```python
from build123d import *

# Parameters (mm, degrees)
F0_R     = 1.5875
F1_DEPTH = 3.048


# Not quite as in the source:
# - a feature names something its author has since deleted; it is built from what else it names


with BuildPart() as f1:
    # F0 (on Front) → F1 (new body)
    with BuildSketch(Plane.XZ):
        with BuildLine():
            Line((-35.5894761368, 60.4198244451), (-34.9866182967, 55.8428987828))
            ThreePointArc((-34.9866182967, 55.8428987828), (-34.9404170511, 56.3828619929), (-34.925, 56.9245788358))
            ThreePointArc((-34.925, 56.9245788358), (-35.092593447, 58.7035019936), (-35.5894761368, 60.4198244451))
        make_face()
        with BuildLine():
            Line((-60.2004882138, 4.1402033601), (-60.2004882138, 8.1089543114))
            ThreePointArc((-60.2004882138, 8.1089543114), (-60.325, 6.1245788358), (-60.2004882138, 4.1402033601))
        make_face()
        with BuildLine():
            ThreePointArc((-34.9866182967, 55.8428987828), (-38.1087610636, 49.8172365933), (-44.45, 47.3995788358))
            Line((-44.45, 47.3995788358), (-44.45, 21.9995788358))
            ThreePointArc((-44.45, 21.9995788358), (-33.9832619763, 18.0603662058), (-28.7109436839, 8.1976758617))
            Line((-28.7109436839, 8.1976758617), (-34.9866182967, 55.8428987828))
        make_face()
        with BuildLine():
            ThreePointArc((-44.45, -9.7504211642), (-54.950325336, -5.7816713228), (-60.2004882138, 4.1402033601))
            Line((-60.2004882138, 4.1402033601), (-54.5067664898, -58.2925744899))
            ThreePointArc((-54.5067664898, -58.2925744899), (-51.9079352447, -50.5666823428), (-44.45, -47.276920164))
            Line((-44.45, -47.276920164), (-44.45, -9.7504211642))
        make_face()
        with BuildLine():
            ThreePointArc((-34.3514989997, -57.3754211642), (-37.3092814629, -50.2347026271), (-44.45, -47.276920164))
            Line((-44.45, -47.276920164), (-44.45, -54.2004211642))
            ThreePointArc((-44.45, -54.2004211642), (-42.2049359697, -55.130357134), (-41.275, -57.3754211642))
            Line((-41.275, -57.3754211642), (-34.3514989997, -57.3754211642))
        make_face()
        with BuildLine():
            Line((-44.45, 21.9995788358), (-44.45, 47.3995788358))
            ThreePointArc((-44.45, 47.3995788358), (-51.5919689055, 50.6223645302), (-53.9009645367, 58.1098612184))
            Line((-53.9009645367, 58.1098612184), (-60.2004882138, 8.1089543114))
            ThreePointArc((-60.2004882138, 8.1089543114), (-54.950325336, 18.0308289943), (-44.45, 21.9995788358))
        make_face()
        with Locations((-48.8420496888, 42.732682374)):
            Circle(F0_R, mode=Mode.SUBTRACT)
        with BuildLine():
            ThreePointArc((-28.7109436839, 8.1976758617), (-33.9832619763, 18.0603662058), (-44.45, 21.9995788358))
            Line((-44.45, 21.9995788358), (-44.45, 9.1638046543))
            ThreePointArc((-44.45, 9.1638046543), (-42.3009428141, 8.2736360216), (-41.4107741814, 6.1245788358))
            ThreePointArc((-41.4107741814, 6.1245788358), (-42.3009428141, 3.9755216499), (-44.45, 3.0853530172))
            Line((-44.45, 3.0853530172), (-44.45, -9.7504211642))
            ThreePointArc((-44.45, -9.7504211642), (-34.1131196636, -5.9238455389), (-28.7595280627, 3.7111341226))
            ThreePointArc((-28.7595280627, 3.7111341226), (-28.6211992399, 4.91433444), (-28.575, 6.1245788358))
            ThreePointArc((-28.575, 6.1245788358), (-28.6090223784, 7.1633535905), (-28.7109436839, 8.1976758617))
        make_face()
        with BuildLine():
            ThreePointArc((-53.9009645367, 58.1098612184), (-51.5919689055, 50.6223645302), (-44.45, 47.3995788358))
            ThreePointArc((-44.45, 47.3995788358), (-38.1087610636, 49.8172365933), (-34.9866182967, 55.8428987828))
            Line((-34.9866182967, 55.8428987828), (-35.5894761368, 60.4198244451))
            ThreePointArc((-35.5894761368, 60.4198244451), (-45.6421147488, 66.37468399), (-53.9009645367, 58.1098612184))
        make_face()
        with BuildLine():
            ThreePointArc((-41.275, 56.9245788358), (-42.2049359697, 54.6795148055), (-44.45, 53.7495788358))
            ThreePointArc((-44.45, 53.7495788358), (-46.6950640303, 59.169642866), (-41.275, 56.9245788358))
        make_face(mode=Mode.SUBTRACT)
        with BuildLine():
            Line((-44.45, 9.1638046543), (-44.45, 21.9995788358))
            ThreePointArc((-44.45, 21.9995788358), (-54.950325336, 18.0308289943), (-60.2004882138, 8.1089543114))
            Line((-60.2004882138, 8.1089543114), (-60.2004882138, 4.1402033601))
            ThreePointArc((-60.2004882138, 4.1402033601), (-54.950325336, -5.7816713228), (-44.45, -9.7504211642))
            Line((-44.45, -9.7504211642), (-44.45, 3.0853530172))
            ThreePointArc((-44.45, 3.0853530172), (-47.4892258186, 6.1245788358), (-44.45, 9.1638046543))
        make_face()
        with BuildLine():
            Line((-7.9375, -57.3754211642), (-34.3514989997, -57.3754211642))
            ThreePointArc((-34.3514989997, -57.3754211642), (-36.803283354, -63.9714386739), (-42.9681138788, -67.3646021105))
            Line((-42.9681138788, -67.3646021105), (-0.5559922874, -65.2934246264))
            ThreePointArc((-0.5559922874, -65.2934246264), (-5.8059062614, -62.7879398695), (-7.9375, -57.3754211642))
        make_face()
        with BuildLine():
            ThreePointArc((-28.7595280627, 3.7111341226), (-34.1131196636, -5.9238455389), (-44.45, -9.7504211642))
            Line((-44.45, -9.7504211642), (-44.45, -47.276920164))
            ThreePointArc((-44.45, -47.276920164), (-37.3092814629, -50.2347026271), (-34.3514989997, -57.3754211642))
            Line((-34.3514989997, -57.3754211642), (-7.9375, -57.3754211642))
            ThreePointArc((-7.9375, -57.3754211642), (-5.6126600757, -51.7627610886), (0, -49.4379211642))
            Line((0, -49.4379211642), (-25.6033683849, -48.186229462))
            ThreePointArc((-25.6033683849, -48.186229462), (-31.1587660622, -45.5255963138), (-33.1463097303, -39.6954091582))
            Line((-33.1463097303, -39.6954091582), (-28.7595280627, 3.7111341226))
        make_face()
        with BuildLine():
            ThreePointArc((-44.45, -47.276920164), (-51.9079352447, -50.5666823428), (-54.5067664898, -58.2925744899))
            ThreePointArc((-54.5067664898, -58.2925744899), (-51.4418867888, -64.6619320978), (-44.9515214608, -67.4614609558))
            Line((-44.9515214608, -67.4614609558), (-42.9681138788, -67.3646021105))
            ThreePointArc((-42.9681138788, -67.3646021105), (-36.803283354, -63.9714386739), (-34.3514989997, -57.3754211642))
            Line((-34.3514989997, -57.3754211642), (-41.275, -57.3754211642))
            ThreePointArc((-41.275, -57.3754211642), (-46.6950640303, -59.6204851945), (-44.45, -54.2004211642))
            Line((-44.45, -54.2004211642), (-44.45, -47.276920164))
        make_face()
        with BuildLine():
            ThreePointArc((0, -49.4379211642), (-5.6126600757, -51.7627610886), (-7.9375, -57.3754211642))
            ThreePointArc((-7.9375, -57.3754211642), (-5.8059062614, -62.7879398695), (-0.5559922874, -65.2934246264))
            Line((-0.5559922874, -65.2934246264), (1.3248513243, -65.2015744479))
            ThreePointArc((1.3248513243, -65.2015744479), (6.0629989954, -62.4983060382), (7.9375, -57.3754211642))
            ThreePointArc((7.9375, -57.3754211642), (5.6126600757, -51.7627610886), (0, -49.4379211642))
        make_face()
        with BuildLine():
            ThreePointArc((3.1965151992, -57.3754211642), (0, -60.5719363635), (-3.1965151992, -57.3754211642))
            ThreePointArc((-3.1965151992, -57.3754211642), (0, -54.178905965), (3.1965151992, -57.3754211642))
        make_face(mode=Mode.SUBTRACT)
    extrude(amount=F1_DEPTH)


solid = f1.part
```
Geometry: final body of the model. Coordinates: model frame, mm. A direction names the side the tool comes from. Coordinates: 2 decimals unless noted, no trailing zeros. Order: outer loops, then holes, each group sorted by start corner. A loop starts at its lowest first (then second) coordinate and runs counter-clockwise, first axis right, second up. Notation, with made-up numbers: M -15,29.25 L 4,29.25 A32 cw 4,61.25 Z; hole C -16.5,77 d5. An arc over 180 degrees is marked long. Answer in a Markdown table with one row per item. Add a question column.
Q1. Section query B-B on x = -11. Return the cut outline in (y, z), and give its area (3 significant figures).
Q2. Mould query, pull axis Z, two halves, no side actions, for faces 3 (the flat face through (-42, -3.048, -14)), 4 (the cylindrical face through (-50.01, -1.5, 43.81)), 5 (the cylindrical face through (-60.325, -1.503, 6.152)). Classes: released by +Z, released by -Z, zero draft, split by the parting line, or undercut.
Q3. Line query: L1, parallel to Z at x = -44.45, y = -2.4; L2, parallel to X at y = -1.5, z = 56; L3, parallel to Z at x = -47, y = -0.65. Output: solid intervals per line, ascending.
Q4. Section query C-C on z = -26. Return the cut outline in (x, y), and give its area (3 significant figures).
Q5. Contact query for a flat-ended pin moving along its axis: P1, Ø1.5, axis at x = -27.5, y = -2.5, coming from the +Z side. Output: stop coordinate, or through.
Q6. Reachability of faces 1 (the cylindrical face through (-31.1, -1.5, -45.59)), 2 (the flat face through (-12.62, -1.5, -48.82)) from +Z, -Z, +X, -X, +Y, -Y: full face, straight path, thin tool, end or side. Return the list, or none.
Q7. Section query A-A on y = -2.5. Count the separate pieces of the cut face and the enclosed holes in it, and give its area (3 significant figures).
Completed:
| question | item | result |
|---|---|---|
| 1 | outline | M -3.05,-65.8 L 0,-65.8 L 0,-48.9 L -3.05,-48.9 Z |
| 1 | area | 51.5 mm2 |
| 2 | face 3 | zero draft |
| 2 | face 4 | undercut |
| 2 | face 5 | split by the parting line |
| 3 | L1 | z = -67.44 to -60.55, -54.2 to 3.09, 9.16 to 53.75, 60.1 to 66.45 |
| 3 | L2 | x = -54.17 to -47.49, -41.41 to -34.97 |
| 3 | L3 | z = -67.15 to -59.27, -55.48 to 4.47, 7.78 to 55.03, 58.82 to 66.1 |
| 4 | outline | M -57.45,-3.05 L -31.76,-3.05 L -31.76,0 L -57.45,0 Z |
| 4 | area | 78.3 mm2 |
| 5 | P1 | stops at z = -47.59 |
| 6 | face 1 | +X, +Y, -Y |
| 6 | face 2 | +Z, +X, +Y, -Y |
| 7 | separate pieces | 1 |
| 7 | enclosed holes | 5 |
| 7 | area | 3,840 mm2 |
